Design review of the part shown in the three views and the two pictorial views. Dimensions are in mm from the part's minimum x, y and z. A direction names the side the tool comes from. Round coordinates to 2 decimals unless told otherwise and drop trailing zeros.
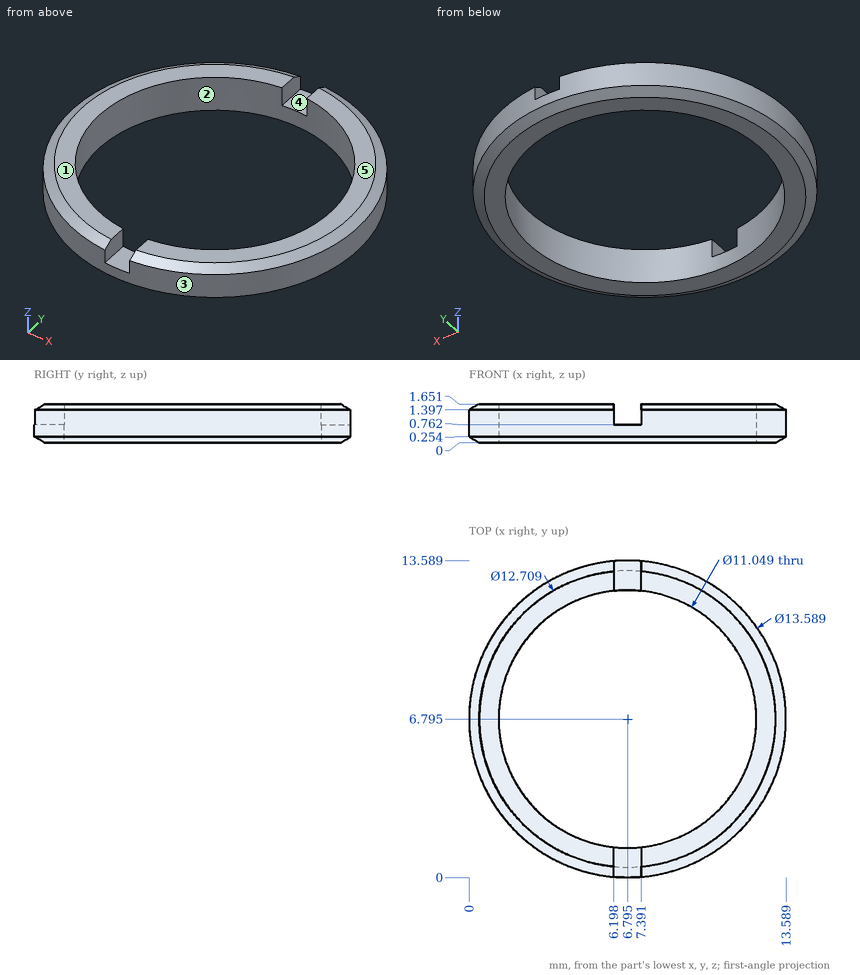
(1) Tool access review of the marked faces 4 and 5: name each direction out of +Z, -Z, +X, -X, +Y, -Y from which nothing blocks a thin tool from reaching the whole face with its end or side.
(2) Draft analysis for pull direction X (two halves, no side actions). For the marked faces 1, 2 and 3, state which applies: pulls with the +X half, pulls with the -X half, needs draft (parallel to the pull), parting line crosses it, or undercut.
(3) Clearance check with flat-ended pins moving along their axes: P1, Ø0.7, axis at y = 0.5, z = 1.5, coming from the +X side (1 decimal); P2, Ø0.7, axis at y = 13, z = 1, coming from the +X side. State where each tip first meets the part, or that it passes through.
(4) Wall thickness on L1, parallel to Y at x = 8.5, z = 0.4; L2, parallel to Y at x = 9.25, z = 0.75 (1 decimal); L3, parallel to X at y = 10.25, z = 0.5 (1 decimal): over which ranges is each line inside the solid? List them lowest first.
Here are the results:
1. face 4: +Z, +Y, -Y
1. face 5: +Z, +X, -X, +Y, -Y
2. face 1: needs draft
2. face 2: undercut
2. face 3: parting line crosses it
3. P1: stops at x = 10.1
3. P2: stops at x = 10.24
4. L1: y = 0.22 to 1.54, 12.05 to 13.37
4. L2: y = 0.5 to 1.8, 11.7 to 13.1
4. L3: x = 0.9 to 2.5, 11.1 to 12.6
